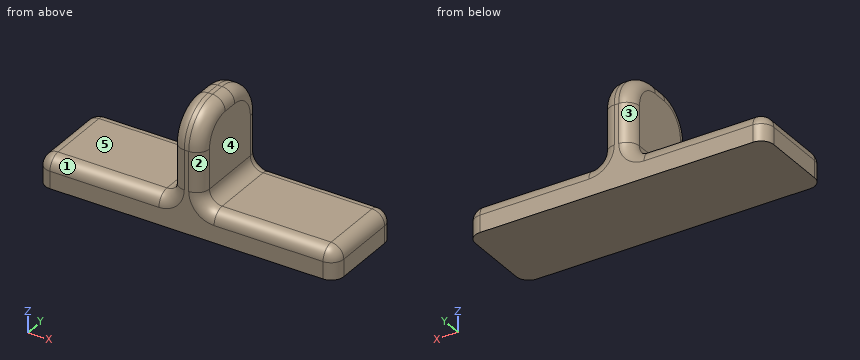
```python
from build123d import *

# Parameters (mm, degrees)
F0_W     = 40
F0_H     = 12
F1_DEPTH = 4
F2_W     = 4
F2_H     = 12
F3_DEPTH = 12
F4_R     = 5
F5_R     = 1.7


with BuildPart() as f1:
    # F0 (on Top) → F1 (new body)
    with BuildSketch(Plane.XY):
        Rectangle(F0_W, F0_H)
    extrude(amount=F1_DEPTH)

    # F2 (on face) → F3 (join)
    with BuildSketch(Plane.XY.offset(4)):
        Rectangle(F2_W, F2_H)
    extrude(amount=F3_DEPTH)

    # F4
    f4_edges = [f1.edges().sort_by_distance(p)[0] for p in [
        (0, -6, 16),
        (0, 6, 16),
    ]]
    fillet(f4_edges, radius=F4_R)

    # F5
    f5_edges = [f1.edges().sort_by_distance(p)[0] for p in [
        (-20, -6, 2),
        (-11, -6, 4),
        (-20, 0, 4),
        (-20, 6, 2),
        (-11, 6, 4),
        (20, -6, 2),
        (20, 6, 2),
        (11, -6, 4),
        (20, 0, 4),
        (11, 6, 4),
        (-2, 6, 7.5),
        (-2, 4.535534, 14.535534),
        (-2, 0, 4),
        (-2, 0, 16),
        (-2, -6, 7.5),
        (-2, -4.535534, 14.535534),
        (2, -6, 7.5),
        (2, 6, 7.5),
        (2, 4.535534, 14.535534),
        (2, 0, 16),
        (2, 0, 4),
    ]]
    fillet(f5_edges, radius=F5_R)


solid = f1.part
```
Geometry: final body of the model. Coordinates: model frame, mm. Face numbers are marked on the shaded views. A direction names the side the tool comes from. Round coordinates to 2 decimals unless told otherwise and drop trailing zeros. Loops run counter-clockwise (first coordinate to the right, second up) from the corner with the lowest first, then second, coordinate; pieces in that order, holes last. Notation, with made-up numbers: (22.5, 48.25) -> (31.5, 48.25) arc R23 ccw to (31.5, 67.25) -> close; hole circle Ø9 at (-26.75, -29.75). An arc over 180 degrees is marked (long way). Write each question's results on one line, items separated by ' | '.
Item 1: Set-up query: the marked faces 1, 2, 3, 4 and 5. Return all of +Z, -Z, +X, -X, +Y, -Y with unobstructed straight access to the full face (end or side cutting, diameter ignored); none if empty.
Answers below:
face 1: +Z, -X, -Y | face 2: +Z, +X, -Y | face 3: +Z, -X, +Y | face 4: +Z, +X, +Y, -Y | face 5: +Z, -X, +Y, -Y
Item 2: Cut plane A-A on z = 8.75. Return the cut outline in (x, y), and give its area (3 significant figures).
Answers below:
outline: (-2, -4.3) arc R1.7 ccw to (-0.3, -6) -> (0.3, -6) arc R1.7 ccw to (2, -4.3) -> (2, 4.3) arc R1.7 ccw to (0.3, 6) -> (-0.3, 6) arc R1.7 ccw to (-2, 4.3) -> close | area: 45.5 mm²
Item 3: Line query: probe 1 along Z at (x, y) = (17.5, 0.5); probe 2 along X at (y, z) = (4, 7.5); probe 3 along X at (y, z) = (4, 14.5). Output: solid intervals per line, ascending. Write a range as [from, to].
Answers below:
probe 1: z = [0, 4] | probe 2: x = [-2, 2] | probe 3: x = [-1.38, 1.38]
Item 4: Cut plane B-B on x = -5.5. Return the cut outline in (y, z).
Answers below:
outline: (-6, 0) -> (6, 0) -> (6, 2.3) arc R1.7 ccw to (4.3, 4) -> (-4.3, 4) arc R1.7 ccw to (-6, 2.3) -> close
Item 5: Pin query (flat end, axial travel): pin 1 Ø4 at (x, y) = (-8.5, -3.5) entering from +Z; pin 2 Ø1 at (x, z) = (-7.5, 4) entering from -Y; pin 3 Ø7 at (y, z) = (0.5, 9) entering from +X. Return the tip coordinate at first contact, or that it passes through.
Answers below:
pin 1: stops at z = 4 | pin 2: stops at y = -5.5 | pin 3: stops at x = 2.01
